Autodesk Inventor part; units mm, degrees
ref_plane "YZ Plane" through (0, 0, 0) normal (1, 0, 0) x (0, 1, 0)
ref_plane "XZ Plane" through (0, 0, 0) normal (0, 1, 0) x (-1, 0, 0)
ref_plane "XY Plane" through (0, 0, 0) normal (0, 0, 1) x (1, 0, 0)
sketch "Sketch1" plane through (0, 0, 0) normal (0, 0, 1) x (1, 0, 0)
  circle A0 centre (0, 0) radius 76.2 construction
  circle A1 centre (0, 0) radius 21.5
  circle A2 centre (0, 0) radius 21.5 construction
  circle A3 centre (0, 0) radius 33.3375
  line L0 (0, 76.2) -> (0, 0) construction
  line L1 (0, 76.2) -> (4.2947, 60.1719)
  line L2 (4.2947, 60.1719) -> (-26.4022, 20.3547)
  circle A4 centre (0, 0) radius 60.325 construction
  arc A5 (30.7227, 63.8735) -> (0, 76.2) centre (0, 31.75) ccw
  line L3 (30.7227, 63.8735) -> (33.309, 1.3784)
  circle A6 centre (0, 0) radius 53.975 construction
  line L4 (27.435, -46.4825) -> (0, 0) construction
  line L5 (27.435, -46.4825) -> (19.5403, -37.2553)
  line L6 (19.5403, -37.2553) -> (30.278, -13.951)
  circle A7 centre (0, 0) radius 42.0688 construction
  arc A8 (-42.2119, -33.6371) -> (27.435, -46.4825) centre (0, 0) ccw
  line L7 (-42.2119, -33.6371) -> (-32.4426, 7.6724)
  line L8 (-42.2119, -33.6371) -> (0, 0) construction
  line L9 (-4.6134, 33.0167) -> (13.0978, 55.9902)
  line L10 (22.8274, 24.296) -> (21.628, 53.2793)
  arc A9 (21.628, 53.2793) -> (13.0978, 55.9902) centre (16.8696, 53.0824) ccw
  line L11 (0, 0) -> (-10.75, 18.6195) construction
  arc A10 (-6.7508, 22.9574) -> (-16.5062, 17.3251) centre (-10.75, 18.6195) ccw
  arc A11 (-17.4815, 12.5159) -> (-16.5062, 17.3251) centre (-22.3601, 16.0087) ccw
  arc A12 (-6.7508, 22.9574) -> (-2.0983, 21.3974) centre (-2.6839, 27.3687) ccw
  arc A13 (16.5062, 17.3251) -> (17.4815, 12.5159) centre (22.3601, 16.0087) ccw
  arc A14 (16.5062, 17.3251) -> (6.7508, 22.9574) centre (10.75, 18.6195) ccw
  arc A15 (2.0983, 21.3974) -> (6.7508, 22.9574) centre (2.6839, 27.3687) ccw
  arc A16 (23.2571, -5.6323) -> (19.5798, -8.8815) centre (25.044, -11.36) ccw
  arc A17 (23.2571, -5.6323) -> (23.2571, 5.6323) centre (21.5, 0) ccw
  arc A18 (19.5798, 8.8815) -> (23.2571, 5.6323) centre (25.044, 11.36) ccw
  arc A19 (6.7508, -22.9574) -> (2.0983, -21.3974) centre (2.6839, -27.3687) ccw
  arc A20 (6.7508, -22.9574) -> (16.5062, -17.3251) centre (10.75, -18.6195) ccw
  arc A21 (17.4815, -12.5159) -> (16.5062, -17.3251) centre (22.3601, -16.0087) ccw
  arc A22 (-16.5062, -17.3251) -> (-17.4815, -12.5159) centre (-22.3601, -16.0087) ccw
  arc A23 (-16.5062, -17.3251) -> (-6.7508, -22.9574) centre (-10.75, -18.6195) ccw
  arc A24 (-2.0983, -21.3974) -> (-6.7508, -22.9574) centre (-2.6839, -27.3687) ccw
  arc A25 (-23.2571, 5.6323) -> (-19.5798, 8.8815) centre (-25.044, 11.36) ccw
  arc A26 (-23.2571, 5.6323) -> (-23.2571, -5.6323) centre (-21.5, 0) ccw
  arc A27 (-19.5798, -8.8815) -> (-23.2571, -5.6323) centre (-25.044, -11.36) ccw
  point P0 (25.3939, -0.9713)
  point P1 (-23.0466, 22.3171)
  point P2 (-2.0983, 21.3974)
  point P3 (2.0983, 21.3974)
  point P4 (17.4815, 12.5159)
  point P5 (19.5798, -8.8815)
  point P6 (2.0983, -21.3974)
  point P7 (-2.0983, -21.3974)
  point P8 (-17.4815, -12.5159)
  point P9 (-19.5798, -8.8815)
  point P10 (-19.5798, 8.8815)
  dimension "d0" = 152.4
  dimension "d14" = 15.875
  dimension "d17" = 84.1375
  dimension "d1" = 43
  dimension "d2" = 43
  dimension "d8" = 66.675
  dimension "d9" = 15
  dimension "d11" = 44.45
  dimension "d12" = 40
  dimension "d15" = 107.95
  dimension "d16" = 10
  dimension "d18" = 30.55
  dimension "d19" = 82
  dimension "d28" = 9.525
  dimension "d29" = 9.525
  dimension "d30" = 4.7625
  dimension "d46" = 11.8
  dimension "d47" = 6
  dimension "d48" = 30
  dimension "d51" = 360
extrude "Extrusion1" add sketch "Sketch1" along normal blind 6.35 contours A3 | A3 L10 A9 L9 L2 L1 A5 L3 | L6 L5 A8 L7 A3
fillet "Fillet1" radius 3.175 4 edges at (19.5403, -37.2553, 3.175) (4.2947, 60.1719, 3.175) (-4.6134, 33.0167, 3.175) (22.8274, 24.296, 3.175)
fillet "Fillet3" radius 3.175 1 edges at (-42.2119, -33.6371, 3.175)
sketch "Sketch2" plane through (0, 0, 6.35) normal (0, 0, 1) x (1, 0, 0)
  arc A0 (30.7227, 63.8735) -> (0, 76.2) centre (0, 31.75) ccw construction
  circle A1 centre (0, 0) radius 76.2 construction
fillet "Fillet4" radius 9.525 1 edges at (30.7227, 63.8735, 3.175)
equation "\"d29\" = d28"
properties part number "Blade" material "Steel, Alloy"
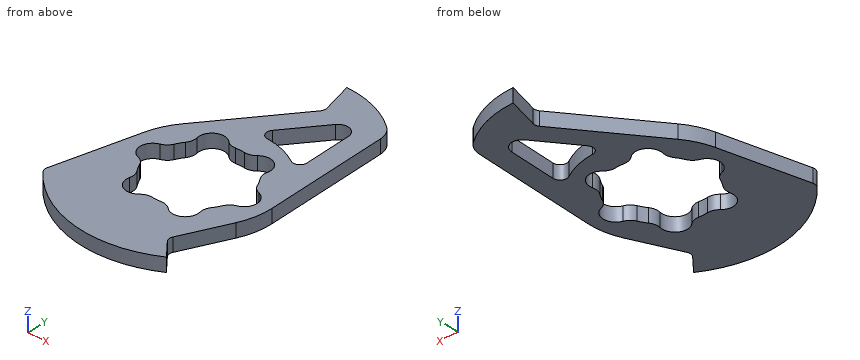
Could you check a few things on this model? Use its own coordinates, in mm. Round coordinates to 2 decimals unless told otherwise and drop trailing zeros. Loops run counter-clockwise (first coordinate to the right, second up) from the corner with the lowest first, then second, coordinate; pieces in that order, holes last. Notation, with made-up numbers: (68.25, 64) -> (96.25, 64) arc R17 cw to (96.25, 83) -> close; hole circle Ø3 at (46, -13). An arc over 180 degrees is marked (long way). Put each result on its own line as item: value.
Q1. I want a section at A-A on y = 35. Write out the boundary of the cut face in (x, z), and give its area (3 significant figures).
Checks:
outline: (-15.11, 0) -> (-0.78, 0) -> (-0.78, 6.35) -> (-15.11, 6.35) -> close; (22.38, 0) -> (31.92, 0) -> (31.92, 6.35) -> (22.38, 6.35) -> close
area: 152 mm2
Q2. I want a section at D-D on z = 1. Give the number of separate pieces and of enclosed holes in the cut face, and give its area (3 significant figures).
Checks:
separate pieces: 1
enclosed holes: 2
area: 4,350 mm2
Q3. For pin 1 Ø8 at (x, y) = (-11, 48.5) entering from +Z; pin 2 Ø3 at (x, z) = (15.5, 3.5) entering from -Y, each with a flat end and sliding along its axis, tell me the tip position at first contact or that it passes through.
Checks:
pin 1: through
pin 2: y = -52.13
Q4. I want a section at C-C on x = -9. Write out the boundary of the cut face in (y, z), and give its area (3 significant figures).
Checks:
outline: (-53.22, 0) -> (-24.25, 0) -> (-24.25, 6.35) -> (-53.22, 6.35) -> close; (24.25, 0) -> (42.93, 0) -> (42.93, 6.35) -> (24.25, 6.35) -> close
area: 303 mm2
Q5. Please list where these lines run through material, in increasing order: line 1 (Y direction, x = 24.5, z = 4.5); line 2 (Y direction, x = 20, z = 1); line 3 (Y direction, x = -6, z = 5.75). Write a range as from..to.
Checks:
line 1: -48.09..-43.05, -26.49..-5.08, 5.08..68.84
line 2: -50.13..-8.11, 8.11..27.84, 56.67..71.45
line 3: -53.64..-22.37, 22.37..46.82
Q6. I want a section at B-B on x = 15. Write out the boundary of the cut face in (y, z), and give its area (3 significant figures).
Checks:
outline: (-51.85, 0) -> (-22.71, 0) -> (-22.71, 6.35) -> (-51.85, 6.35) -> close; (22.71, 0) -> (29.77, 0) -> (29.77, 6.35) -> (22.71, 6.35) -> close; (57.46, 0) -> (73.59, 0) -> (73.59, 6.35) -> (57.46, 6.35) -> close
area: 332 mm2
